```python
from build123d import *

# Parameters (mm, degrees)
SKETCH_1_R          = 2.6
SKETCH_1_R_2        = 6.1
EXTRUDE_1_DEPTH     = 9
CUT_EXTRUDE_START   = -10
SKETCH_2_R          = 3.4
SKETCH_2_R_2        = 2.6
CUT_EXTRUDE_1_DEPTH = 10


with BuildPart() as part:
    # 草图1 → 凸台-拉伸1 (new body)
    with BuildSketch(Plane(origin=(0, 0, 0), x_dir=(1, 0, 0), z_dir=(0, 1, 0))):
        with BuildLine():
            ThreePointArc((10.005741881, 19.864209328), (9.487119891, 20.17017771), (8.962832505, 20.466333337))
            Line((8.962832505, 20.466333337), (-13.385709221, -0.397651364))
            ThreePointArc((-13.385709221, -0.397651364), (-16.561513437, -7.747050572), (-13.327428101, -15.070990303))
            Line((-13.327428101, -15.070990303), (5.481515962, -32.352919827))
            ThreePointArc((5.481515962, -32.352919827), (5.510229247, -32.338868299), (5.538926138, -32.32478332))
            ThreePointArc((5.538926138, -32.32478332), (7.091187682, -34.107638735), (8.962832505, -35.551603759))
            ThreePointArc((8.962832505, -35.551603759), (9.487119891, -35.255448132), (10.005741881, -34.94947975))
            ThreePointArc((10.005741881, -34.94947975), (9.684229712, -32.57790044), (8.898482853, -30.317289822))
            ThreePointArc((8.898482853, -30.317289822), (9.650626544, -29.789793539), (10.384730504, -29.237467697))
            ThreePointArc((10.384730504, -29.237467697), (12.29188983, -30.683324466), (14.448043063, -31.721959019))
            ThreePointArc((14.448043063, -31.721959019), (14.899299295, -31.323269626), (15.342973746, -30.916159812))
            ThreePointArc((15.342973746, -30.916159812), (14.535408326, -28.663251339), (13.296824545, -26.615406445))
            ThreePointArc((13.296824545, -26.615406445), (13.922859447, -25.943057755), (14.526086474, -25.250172762))
            ThreePointArc((14.526086474, -25.250172762), (16.692180319, -26.267913372), (19.017160696, -26.835561803))
            ThreePointArc((19.017160696, -26.835561803), (19.375663711, -26.351763284), (19.724999921, -25.861304691))
            ThreePointArc((19.724999921, -25.861304691), (18.466675733, -23.825529966), (16.829387085, -22.079951444))
            ThreePointArc((16.829387085, -22.079951444), (17.30195247, -21.292135211), (17.747938649, -20.488973466))
            ThreePointArc((17.747938649, -20.488973466), (20.078298317, -21.034117768), (22.47049304, -21.105971118))
            ThreePointArc((22.47049304, -21.105971118), (22.720574536, -20.558207789), (22.960304836, -20.005835811))
            ThreePointArc((22.960304836, -20.005835811), (21.306216685, -18.276167958), (19.34178054, -16.909145965))
            ThreePointArc((19.34178054, -16.909145965), (19.640223033, -16.040293539), (19.909476627, -15.161957065))
            ThreePointArc((19.909476627, -15.161957065), (22.302254219, -15.210679637), (24.657112899, -14.783597569))
            ThreePointArc((24.657112899, -14.783597569), (24.787843115, -14.195809317), (24.907490141, -13.60566526))
            ThreePointArc((24.907490141, -13.60566526), (22.929929617, -12.257699063), (20.724201261, -11.328979021))
            ThreePointArc((20.724201261, -11.328979021), (20.835477492, -10.417063422), (20.916230828, -9.501939738))
            ThreePointArc((20.916230828, -9.501939738), (23.266850481, -9.052111169), (25.481454494, -8.14475922))
            ThreePointArc((25.481454494, -8.14475922), (25.487119891, -7.542635211), (25.481454494, -6.940511202))
            ThreePointArc((25.481454494, -6.940511202), (23.266850481, -6.033159253), (20.916230828, -5.583330684))
            ThreePointArc((20.916230828, -5.583330684), (20.835477492, -4.668206999), (20.724201261, -3.7562914))
            ThreePointArc((20.724201261, -3.7562914), (22.929929617, -2.827571359), (24.907490141, -1.479605162))
            ThreePointArc((24.907490141, -1.479605162), (24.787843115, -0.889461105), (24.657112899, -0.301672852))
            ThreePointArc((24.657112899, -0.301672852), (22.302254219, 0.125409215), (19.909476627, 0.076686643))
            ThreePointArc((19.909476627, 0.076686643), (19.640223033, 0.955023117), (19.34178054, 1.823875544))
            ThreePointArc((19.34178054, 1.823875544), (21.306216685, 3.190897536), (22.960304836, 4.92056539))
            ThreePointArc((22.960304836, 4.92056539), (22.720574536, 5.472937368), (22.47049304, 6.020700696))
            ThreePointArc((22.47049304, 6.020700696), (20.078298317, 5.948847346), (17.747938649, 5.403703045))
            ThreePointArc((17.747938649, 5.403703045), (17.30195247, 6.206864789), (16.829387085, 6.994681022))
            ThreePointArc((16.829387085, 6.994681022), (18.466675733, 8.740259544), (19.724999921, 10.77603427))
            ThreePointArc((19.724999921, 10.77603427), (19.375663711, 11.266492862), (19.017160696, 11.750291382))
            ThreePointArc((19.017160696, 11.750291382), (16.692180319, 11.18264295), (14.526086474, 10.16490234))
            ThreePointArc((14.526086474, 10.16490234), (13.922859447, 10.857787333), (13.296824545, 11.530136023))
            ThreePointArc((13.296824545, 11.530136023), (14.535408326, 13.577980918), (15.342973746, 15.830889391))
            ThreePointArc((15.342973746, 15.830889391), (14.899299295, 16.237999204), (14.448043063, 16.636688597))
            ThreePointArc((14.448043063, 16.636688597), (12.29188983, 15.598054044), (10.384730504, 14.152197275))
            ThreePointArc((10.384730504, 14.152197275), (9.650626544, 14.704523117), (8.898482853, 15.2320194))
            ThreePointArc((8.898482853, 15.2320194), (9.684229712, 17.492630019), (10.005741881, 19.864209328))
        make_face()
        with Locations(Location((6.745512081, -19.072672674, 0), (0, 0, 270))):
            Circle(SKETCH_1_R, mode=Mode.SUBTRACT)
        with Locations(Location((8.35961056, 1.436393055, 0), (0, 0, 270))):
            Circle(SKETCH_1_R, mode=Mode.SUBTRACT)
        with Locations(Location((-6.561592317, -7.707331828, 0), (0, 0, 270))):
            Circle(SKETCH_1_R_2, mode=Mode.SUBTRACT)
    extrude(amount=EXTRUDE_1_DEPTH)

    # 草图2 → 切除-拉伸1 (cut)
    # profile 1 of 2: a face of its own
    with BuildSketch(Plane(origin=(0, 9, 0), x_dir=(1, 0, 0), z_dir=(0, 1, 0)).offset(CUT_EXTRUDE_START)):
        with Locations(Location((8.35961056, 1.436393055, 0), (0, 0, 270))):
            Circle(SKETCH_2_R)
        with Locations((8.35961056, 1.436393055)):
            Circle(SKETCH_2_R_2, mode=Mode.SUBTRACT)
    # profile 2 of 2: a face of its own
    with BuildSketch(Plane(origin=(0, 9, 0), x_dir=(1, 0, 0), z_dir=(0, 1, 0)).offset(CUT_EXTRUDE_START)):
        with Locations(Location((6.745512081, -19.072672674, 0), (0, 0, 270))):
            Circle(SKETCH_2_R)
        with Locations((6.745512081, -19.072672674)):
            Circle(SKETCH_2_R_2, mode=Mode.SUBTRACT)
    extrude(amount=CUT_EXTRUDE_1_DEPTH, mode=Mode.SUBTRACT)


solid = part.part
```
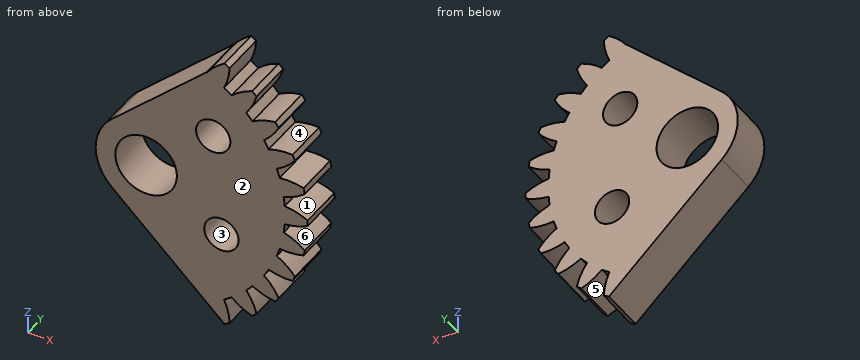
Could you check a few things on this model? Use its own coordinates, in mm. Face numbers are marked on the shaded views. A direction names the side the tool comes from. Coordinates: 2 decimals unless noted, no trailing zeros. Loops run counter-clockwise (first coordinate to the right, second up) from the corner with the lowest first, then second, coordinate; pieces in that order, holes last.
1) Imagine slicing it at C-C (y = 7.5). State how many separate pieces and enclosed holes the cut face has, and give its area (3 significant figures).
Reported:
separate pieces: 1
enclosed holes: 3
area: 1,140 mm2
2) Please list where these lines run through material, in increasing order: line 1 along Z through (x, y) = (6, 7.5); line 2 along X through (y, z) = (2.5, 7.5); line 3 along Z through (x, y) = (18.5, 2.25).
Reported:
line 1: z = -17.7 to -3.88, 1.01 to 15.76, 22.39 to 32.93
line 2: x = -16.56 to -12.66, -0.47 to 25.49
line 3: z = -11.67 to -8.78, -5.63 to 20.72, 23.87 to 26.75
3) Thinking about a two-plate mould opening in X: for the marked faces 1, 2 and 3, which applies, released by +X, released by -X, zero draft, split by the parting line, or undercut?
Reported:
face 1: released by +X
face 2: zero draft
face 3: undercut
4) Imagine slicing it at A-A (x = 21.5). List the corners of the cut face in (y, z) for me, and give its area (3 significant figures).
Reported:
outline: (0, -6.05) - (9, -6.05) - (9, -3.36) - (0, -3.36) - close; (0, -0.16) - (9, -0.16) - (9, 3.49) - (0, 3.49) - close; (0, 5.65) - (9, 5.65) - (9, 9.44) - (0, 9.44) - close; (0, 11.6) - (9, 11.6) - (9, 15.25) - (0, 15.25) - close; (0, 18.45) - (9, 18.45) - (9, 21.13) - (0, 21.13) - close
area: 148 mm2
5) Will these pins go through, and if not, where does the flat tip stop? pin 1 Ø4 at (y, z) = (3, 19) entering from +X; pin 2 Ø1 at (y, z) = (5.5, 0.5) entering from +X; pin 3 Ø5 at (x, y) = (-1, 4) entering from +Z.
Reported:
pin 1: stops at x = 22.96
pin 2: stops at x = 24.81
pin 3: stops at z = 28.69
6) Imagine slicing it at D-D (z = -13.5). List the corners of the cut face in (x, y) for me.
Reported:
outline: (1.5, 0) - (14.5, 0) - (14.5, 9) - (1.5, 9) - close
7) Which directions (+Z, -Z, +X, -X, +Y, -Y) give clear straight access to the entire face, cutting with the end or side of a thin tool? Please do the marked faces 4, 5 and 6.
Reported:
face 4: +Y, -Y
face 5: -Z, +Y, -Y
face 6: +X, +Y, -Y
8) Imagine slicing it at B-B (x = -3.5). List the corners of the cut face in (y, z) for me.
Reported:
outline: (0, -8.83) - (9, -8.83) - (9, 2.43) - (0, 2.43) - close; (0, 12.98) - (9, 12.98) - (9, 24.1) - (0, 24.1) - close
